Could you check a few things on this drawing? It's one solid part, dimensions in mm from its lowest x, y, z. A direction names the side the tool comes from. Coordinates: 2 decimals unless noted, no trailing zeros. Order: outer loops, then holes, each group sorted by start corner. A loop starts at its lowest first (then second) coordinate and runs counter-clockwise, first axis right, second up. Notation, with made-up numbers: (28.25, 55.25) - (44.25, 55.25) arc R21 cw to (44.25, 88.25) - close; hole circle Ø5 at (86.5, 59). An arc over 180 degrees is marked (long way). Answer in a Markdown table with one row per item. Add a question column.
Item 1: I want a section at A-A (x = 35). Please give me the cut outline in (y, z).
Item 2: If I drill on line 1 along Y through (x, z) = (35, 6); line 2 along Z through (x, y) = (28, 9.5); line 3 along Y through (x, z) = (37, 2.5), over which ranges is the centre line in solid material (lowest first)? Write a range as from..to.
Item 3: On a 3-axis mill with a long thin cutter (end or side, diameter ignored), from which of +Z, -Z, +X, -X, +Y, -Y can I reach the whole of each face in a straight line? I mean the marked faces 4 and 5. Say none if no direction works.
Item 4: I want a section at C-C (z = 5.5). Please give me the cut outline in (x, y).
Item 5: Will these pins go through, and if not, where does the flat tip stop? pin 1 Ø1 at (x, y) = (10.5, 48) entering from +Z; pin 2 Ø4 at (x, y) = (28, 54.5) entering from -Z; pin 3 Ø1.5 at (x, z) = (26, 3.5) entering from +Y; pin 4 Ø3 at (x, z) = (7, 2) entering from +Y.
Item 6: Thinking about a two-plate mould opening in Y: for the marked faces 1, 2 and 3, which applies, +Y half, -Y half, draft (parallel to the pull), parting line (faces both ways), or undercut?
Item 7: I want a section at D-D (y = 49.5). Please give me the cut outline in (x, z).
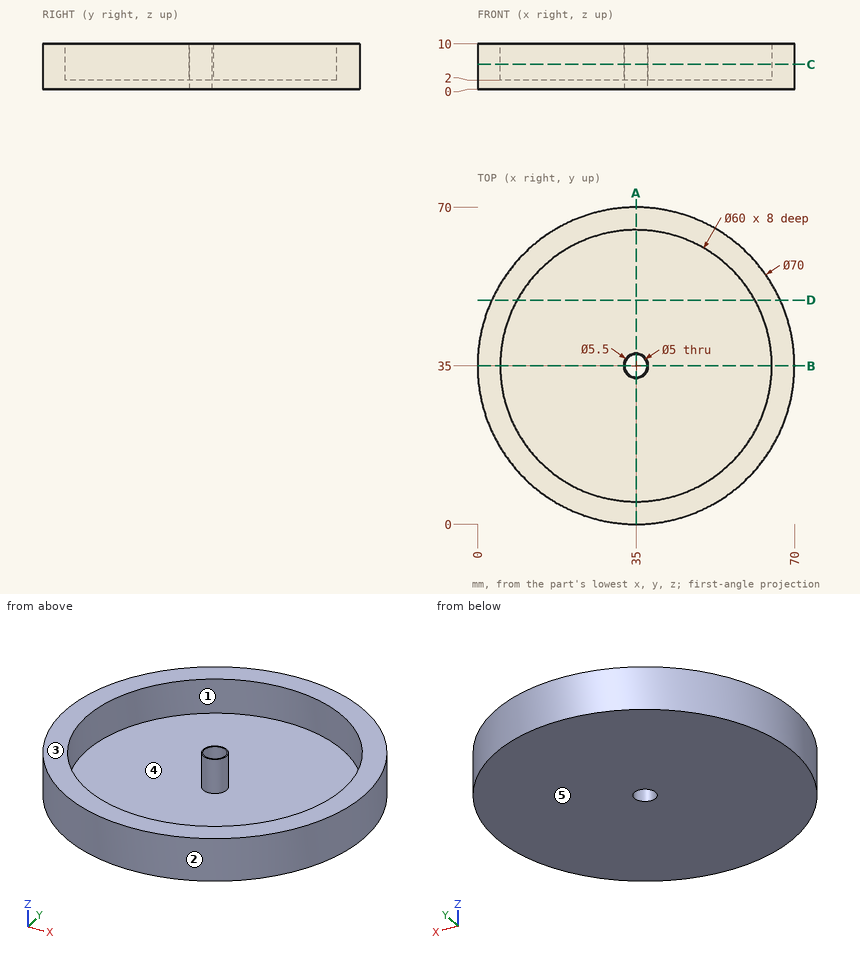
Values follow:
| question | item | result |
|---|---|---|
| 1 | outline | (0, 0) - (32.5, 0) - (32.5, 10) - (32.25, 10) - (32.25, 2) - (5, 2) - (5, 10) - (0, 10) - close; (37.5, 0) - (70, 0) - (70, 10) - (65, 10) - (65, 2) - (37.75, 2) - (37.75, 10) - (37.5, 10) - close |
| 2 | line 1 | y = 0..5, 32.25..32.5, 37.5..37.75, 65..70 |
| 2 | line 2 | z = 0..2 |
| 2 | line 3 | y = 0.06..5.07, 33.11..33.5, 36.5..36.89, 64.93..69.94 |
| 3 | face 4 | +Z |
| 3 | face 5 | -Z, +X, -X, +Y, -Y |
| 4 | outline | circle Ø70 at (35, 35); circle Ø5.5 at (35, 35); hole circle Ø60 at (35, 35); hole circle Ø5 at (35, 35) |
| 5 | pin 1 | stops at z = 2 |
| 5 | pin 2 | stops at z = 0 |
| 5 | pin 3 | stops at y = 69.01 |
| 5 | pin 4 | stops at y = 57.86 |
| 6 | face 1 | undercut |
| 6 | face 2 | parting line |
| 6 | face 3 | draft |
| 7 | outline | (3.14, 0) - (66.86, 0) - (66.86, 10) - (61.26, 10) - (61.26, 2) - (8.74, 2) - (8.74, 10) - (3.14, 10) - close |
